Geometry: final body of the model. Coordinates: model frame, mm. Give positions to 0.01 mm unless a question says otherwise; leave off trailing zeros. Loops run counter-clockwise (first coordinate to the right, second up) from the corner with the lowest first, then second, coordinate; pieces in that order, holes last. Notation, with made-up numbers: (36, 25) -> (92, 25) arc R28 ccw to (92, 60) -> close; hole circle Ø7 at (83.25, 47). An arc over 180 degrees is marked (long way). Answer in a Markdown table with one row per item. Add a question column.
1) Section query B-B (z = 314.5). Return the cut outline in (x, y), plus the area to 3 significant figures.
2) Line query: line 1 (X direction, y = -6, z = 376); line 2 (Z direction, x = -63, y = 4); line 3 (Y direction, x = -39, z = -261.5). Output: solid intervals per line, ascending. Write a range as from..to.
3) Section query A-A (y = 17). Return the cut outline in (x, z).
4) First-contact query: P1, Ø15, axis at x = -50.5, z = 153.5, coming from the +Y side. Flat tip, straight axial feed; report the tip coordinate or a pass-through.
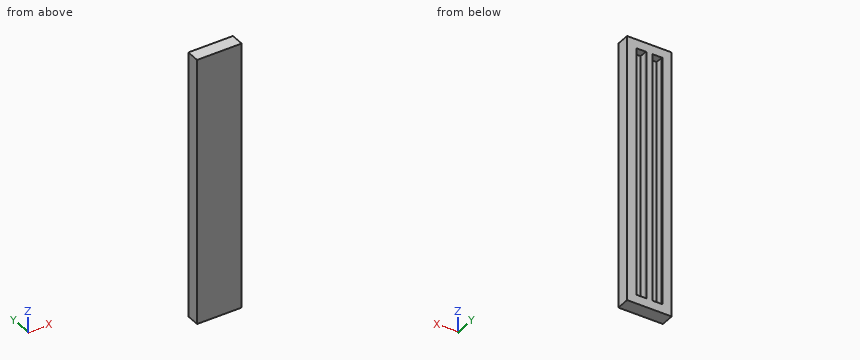
```python
from build123d import *

# Parameters (mm, degrees)
SKETCH1_W           = 250
SKETCH1_H           = 75
BOSS_EXTRUDE1_DEPTH = 750
SKETCH2_W           = 50
SKETCH2_H           = 45
CUT_EXTRUDE1_DEPTH  = 700
FILLET1_R           = 5


with BuildPart() as part:
    # Sketch1 → Boss-Extrude1 (new, symmetric)
    with BuildSketch(Plane.XY):
        Rectangle(SKETCH1_W, SKETCH1_H)
    extrude(amount=BOSS_EXTRUDE1_DEPTH, both=True)

    # Sketch2 → Cut-Extrude1 (cut, symmetric)
    with BuildSketch(Plane.XY):
        with Locations((-45, 15)):
            Rectangle(SKETCH2_W, SKETCH2_H)
        with Locations((45, 15)):
            Rectangle(SKETCH2_W, SKETCH2_H)
    extrude(amount=CUT_EXTRUDE1_DEPTH, both=True, mode=Mode.SUBTRACT)

    # Fillet1
    fillet1_edges = [part.edges().sort_by_distance(p)[0] for p in [
        (-70, 37.5, 0),
        (-20, 37.5, 0),
        (20, 37.5, 0),
        (70, 37.5, 0),
    ]]
    fillet(fillet1_edges, radius=FILLET1_R)


solid = part.part
```
Evaluation:
| question | item | result |
|---|---|---|
| 1 | outline | (-125, -37.5) -> (125, -37.5) -> (125, 37.5) -> (75, 37.5) arc R5 ccw to (70, 32.5) -> (70, -7.5) -> (20, -7.5) -> (20, 32.5) arc R5 ccw to (15, 37.5) -> (-15, 37.5) arc R5 ccw to (-20, 32.5) -> (-20, -7.5) -> (-70, -7.5) -> (-70, 32.5) arc R5 ccw to (-75, 37.5) -> (-125, 37.5) -> close |
| 1 | area | 14,200 mm² |
| 2 | line 1 | -125..-70, -20..20, 70..125 |
| 2 | line 2 | -750..-700, 700..750 |
| 2 | line 3 | -37.5..-7.5 |
| 3 | outline | (-125, -750) -> (125, -750) -> (125, 750) -> (-125, 750) -> close; hole (-70, -700) -> (-20, -700) -> (-20, 700) -> (-70, 700) -> close; hole (20, -700) -> (70, -700) -> (70, 700) -> (20, 700) -> close |
| 4 | P1 | y = -7.5 |
